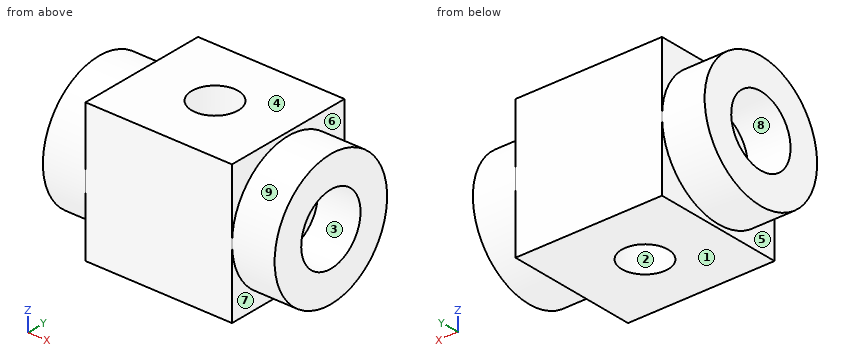
from build123d import *

# Parameters (mm, degrees)
SKETCH1_W           = 31.6
SKETCH1_H           = 28.428065026
BOSS_EXTRUDE1_DEPTH = 30
SKETCH2_R           = 14.214032513
BOSS_EXTRUDE2_DEPTH = 25
SKETCH3_R           = 7.5
CUT_EXTRUDE1_DEPTH  = 75
SKETCH4_R           = 5
CUT_EXTRUDE2_DEPTH  = 75
BOSS_EXTRUDE3_REACH = 30.428
SKETCH5_W           = 4.702962509
SKETCH5_H           = 30
SKETCH5_W_2         = 4.693068718


with BuildPart() as part:
    # Sketch1 → Boss-Extrude1 (new body)
    with BuildSketch(Plane.XY):
        Rectangle(SKETCH1_W, SKETCH1_H)
    extrude(amount=BOSS_EXTRUDE1_DEPTH)

    # Sketch2 → Boss-Extrude2 (add, symmetric)
    with BuildSketch(Plane(origin=(0, 0, 0), x_dir=(0, 0, -1), z_dir=(1, 0, 0))):
        with Locations((-15, 0)):
            Circle(SKETCH2_R)
    extrude(amount=BOSS_EXTRUDE2_DEPTH, both=True)

    # Sketch3 → Cut-Extrude1 (cut)
    with BuildSketch(Plane(origin=(25, 0, 0), x_dir=(0, 0, -1), z_dir=(1, 0, 0))):
        with Locations((-15, 0)):
            Circle(SKETCH3_R)
    extrude(amount=-CUT_EXTRUDE1_DEPTH, mode=Mode.SUBTRACT)

    # Sketch4 → Cut-Extrude2 (cut)
    with BuildSketch(Plane(origin=(0, 0, 0), x_dir=(-1, 0, 0), z_dir=(0, 0, -1))):
        Circle(SKETCH4_R)
    extrude(amount=-CUT_EXTRUDE2_DEPTH, mode=Mode.SUBTRACT)

    # Sketch5 → Boss-Extrude3 (add, up to next)
    with BuildSketch(Plane(origin=(0, 14.214032513, 0), x_dir=(1, 0, 0), z_dir=(0, 1, 0)), mode=Mode.PRIVATE) as boss_extrude3_sk1:
        with Locations((-13.448518745, -15)):
            Rectangle(SKETCH5_W, SKETCH5_H)
    boss_extrude3_tool1 = extrude(boss_extrude3_sk1.sketch, amount=-BOSS_EXTRUDE3_REACH, mode=Mode.PRIVATE) - part.part
    add(boss_extrude3_tool1.solids().sort_by_distance((-13.448519, 14.214033, 15))[0])
    # Sketch5 → Boss-Extrude3 (add, up to next)
    with BuildSketch(Plane(origin=(0, 14.214032513, 0), x_dir=(1, 0, 0), z_dir=(0, 1, 0)), mode=Mode.PRIVATE) as boss_extrude3_sk2:
        with Locations((13.453465641, -15)):
            Rectangle(SKETCH5_W_2, SKETCH5_H)
    boss_extrude3_tool2 = extrude(boss_extrude3_sk2.sketch, amount=-BOSS_EXTRUDE3_REACH, mode=Mode.PRIVATE) - part.part
    add(boss_extrude3_tool2.solids().sort_by_distance((13.453466, 14.214033, 15))[0])


solid = part.part
Design review of the part built by this model. Coordinates are the model's own, in mm. Face numbers are marked on the shaded views. A direction names the side the tool comes from. Give positions to 0.01 mm unless a question says otherwise; leave off trailing zeros. Loops run counter-clockwise (first coordinate to the right, second up) from the corner with the lowest first, then second, coordinate; pieces in that order, holes last. Notation, with made-up numbers: (34.5, -37.75) - (44.5, -37.75) arc R9 cw to (44.5, -23.75) - close; hole circle Ø6 at (-40, 45). An arc over 180 degrees is marked (long way). Use CSV: the item, a comma, the result in double quotes. Start each with the question number.
1. Insertion check: P1, Ø4.5, axis at y = -3, z = 15, coming from the +X side; P2, Ø2, axis at y = -1.5, z = 16.5, coming from the -X side; P3, Ø16, axis at x = 0, y = 0, coming from the -Z side. Each pin has a flat end and moves straight along its axis. Give the tip position at first contact, or say it passes through.
2. Wall thickness on L1, parallel to X at y = 1.5, z = 18.5; L2, parallel to Y at x = 0, z = 3; L3, parallel to Y at x = -4, z = 15: over which ranges is each line inside the solid? List them lowest first.
3. Add section B-B (x = 0). State the section outline as (y, z) points, plus the area to 3 significant figures.
4. Machinability: for the marked faces 5, 6, 7, 8 and 9, which of the approach directions +Z, -Z, +X, -X, +Y, -Y give a long, thin tool a straight path to every point of the face, cutting with its end or side? Answer none if there is none.
5. Draft analysis for pull direction Z (two halves, no side actions). For the marked faces 1, 2, 3 and 4, state which applies: released by +Z, released by -Z, zero draft, split by the parting line, or undercut.
6. Add section D-D (x = 9). State the section outline as (y, z) points.
7. Add section C-C (z = 6). State the section outline as (x, y) points, plus the area to 3 significant figures.
Results found:
1,P1,"stops at x = 15.8"
1,P2,"stops at x = -15.8"
1,P3,"stops at z = 0"
2,L1,"x = -15.8 to -11.1, 11.11 to 15.8"
2,L2,"y = -14.21 to -5, 5 to 14.21"
2,L3,"y = -14.21 to -7.5, 7.5 to 14.21"
3,outline,"(-14.21, 0) - (-5, 0) - (-5, 9.41) arc R7.5 cw to (-5, 20.59) - (-5, 30) - (-14.21, 30) - close; (5, 0) - (14.21, 0) - (14.21, 30) - (5, 30) - (5, 20.59) arc R7.5 cw to (5, 9.41) - close"
3,area,"514 mm²"
4,face 5,"-Z, -X"
4,face 6,"+Z, +X"
4,face 7,"-Z, +X"
4,face 8,"-X"
4,face 9,"+X"
5,face 1,"released by -Z"
5,face 2,"zero draft"
5,face 3,"undercut"
5,face 4,"released by +Z"
6,outline,"(-14.21, 0) - (14.21, 0) - (14.21, 30) - (-14.21, 30) - close; hole circle Ø15 at (0, 15)"
7,outline,"(-25, -11) - (-15.8, -11) - (-15.8, -14.21) - (15.8, -14.21) - (15.8, -11) - (25, -11) - (25, 11) - (15.8, 11) - (15.8, 14.21) - (-15.8, 14.21) - (-15.8, 11) - (-25, 11) - close; hole circle Ø10 at (0, 0)"
7,area,"1,220 mm²"
